```python
from build123d import *

# Parameters (mm, degrees)
SKETCH_1_W               = 35
SKETCH_1_H               = 40
EXTRUDE_1_DEPTH          = 2
SKETCH_2_R               = 1.6
CUT_EXTRUDE_1_DEPTH      = 2
SKETCH_3_W               = 6
SKETCH_3_H               = 6
EXTRUDE_2_DEPTH          = 22
SKETCH_4_W               = 32
SKETCH_4_H               = 32
SKETCH_4_R               = 1.65
EXTRUDE_3_DEPTH          = 3
SKETCH_5_W               = 2.5
SKETCH_5_H               = 22
EXTRUDE_4_DEPTH          = 3
PATTERN_CIRCULAR_1_COUNT = 4


with BuildPart() as part:
    # 草图1 → 凸台-拉伸1 (new body)
    with BuildSketch(Plane(origin=(0, 0, 0), x_dir=(1, 0, 0), z_dir=(0, 1, 0))):
        Rectangle(SKETCH_1_W, SKETCH_1_H)
    extrude(amount=EXTRUDE_1_DEPTH)

    # 草图2 → 切除-拉伸1 (cut)
    with BuildSketch(Plane(origin=(0, 2, 0), x_dir=(1, 0, 0), z_dir=(0, 1, 0))):
        with Locations(Location((-12.5, 15, 0), (0, 0, 270))):
            Circle(SKETCH_2_R)
        with Locations(Location((12.5, 15, 0), (0, 0, 90))):
            Circle(SKETCH_2_R)
        with Locations(Location((12.5, -15, 0), (0, 0, 270))):
            Circle(SKETCH_2_R)
        with Locations(Location((-12.5, -15, 0), (0, 0, 90))):
            Circle(SKETCH_2_R)
    extrude(amount=-CUT_EXTRUDE_1_DEPTH, mode=Mode.SUBTRACT)

    # 草图3 → 凸台-拉伸2 (add)
    with BuildSketch(Plane(origin=(0, 2, 0), x_dir=(1, 0, 0), z_dir=(0, 1, 0))):
        Rectangle(SKETCH_3_W, SKETCH_3_H)
    extrude(amount=EXTRUDE_2_DEPTH)

    # 草图4 → 凸台-拉伸3 (add)
    with BuildSketch(Plane(origin=(0, 24, 0), x_dir=(1, 0, 0), z_dir=(0, 1, 0))):
        Rectangle(SKETCH_4_W, SKETCH_4_H)
        with Locations(Location((-7.78, 7.78, 0), (0, 0, 270))):
            Circle(SKETCH_4_R, mode=Mode.SUBTRACT)
        with Locations(Location((7.78, 7.78, 0), (0, 0, 90))):
            Circle(SKETCH_4_R, mode=Mode.SUBTRACT)
        with Locations(Location((7.78, -7.78, 0), (0, 0, 270))):
            Circle(SKETCH_4_R, mode=Mode.SUBTRACT)
        with Locations(Location((-7.78, -7.78, 0), (0, 0, 90))):
            Circle(SKETCH_4_R, mode=Mode.SUBTRACT)
    extrude(amount=EXTRUDE_3_DEPTH)

    # 草图5 → 凸台-拉伸4 (add)
    with BuildSketch(Plane.XY.offset(3)):
        with Locations((0, 13)):
            Rectangle(SKETCH_5_W, SKETCH_5_H)
    extrude_4 = extrude(amount=EXTRUDE_4_DEPTH)

    # 阵列(圆周)1: 凸台-拉伸4 ×4 about axis
    pattern_circular_1_axis = Axis((0, 0, 0), (0, 1, 0))
    for i in range(1, PATTERN_CIRCULAR_1_COUNT):
        add(extrude_4.rotate(pattern_circular_1_axis, i * 360 / PATTERN_CIRCULAR_1_COUNT))


solid = part.part
```
Geometry check sheet. Reference: the model listing, model coordinates, mm. A direction names the side the tool comes from. Coordinates: 2 decimals unless noted, no trailing zeros. Order: outer loops, then holes, each group sorted by start corner. A loop starts at its lowest first (then second) coordinate and runs counter-clockwise, first axis right, second up. Notation, with made-up numbers: M 42,-34.75 L 71,-34.75 A29 cw 71,-5.75 Z; hole C 15,-8.5 d3. An arc over 180 degrees is marked long. One line per question, with ' | ' between items. Start each with the question number.
Item 1: Set-up check for faces 4 (the flat face through (-4, 13, 1.25)), 5 (the flat face through (-3, 13, -2)), 6 (the flat face through (1.25, 13, 4)), 7 (the cylindrical face through (12.43, 1.01, -13.4)), 8 (the cylindrical face through (-9.4, 25.5, -8.1)): record each of +Z, -Z, +X, -X, +Y, -Y from which the full face is reachable in a straight line by a thin tool's end or side.
Item 2: Gauge pin test, flat ends, axial feed: pin 1 (0.9 mm diameter, centred on y = 18.5, z = 2.5, fed in from +X); pin 2 (0.9 mm diameter, centred on x = 2.5, y = 14.5, fed in from -Z); pin 3 (1.5 mm diameter, centred on x = -5, y = 25, fed in from -Z). Record the tip position at first contact, or that the pin passes through.
Item 3: Cross-section at A-A on z = -12. Enter the section's corners in (x, y).
Item 4: Cross-section at C-C on z = -7.78. Enter the section's corners in (x, y).
Item 5: Cross-section at D-D on x = -5.5. Enter the section's corners in (y, z).
Item 6: Cross-section at B-B on x = -12.5. Enter the section's corners in (y, z).
Item 7: Draft check along X on faces 1 (the cylindrical face through (-13.58, 1.01, 16.18)), 2 (the flat face through (-4, 13, -1.25)), 3 (the flat face through (3, 13, -2)). Enter one of: pulls with the +X half, pulls with the -X half, needs draft (parallel to the pull), parting line crosses it, or undercut.
Item 8: Material ranges on L1, parallel to X at y = 25.85, z = 7.78; L2, parallel to X at y = 0.6, z = 15; L3, parallel to Y at x = -1, z = -7, recorded low to high. Write a range as [from, to].
Findings:
1) face 4: +Z, -X | face 5: -Z, -X | face 6: +Z, +X | face 7: -Y | face 8: +Y
2) pin 1: stops at x = 3 | pin 2: stops at z = -3 | pin 3: stops at z = -16
3) outline: M -17.5,0 L 17.5,0 L 17.5,2 L -17.5,2 Z; M -16,24 L 16,24 L 16,27 L -16,27 Z
4) outline: M -17.5,0 L 17.5,0 L 17.5,2 L -17.5,2 Z; M -16,24 L -9.43,24 L -9.43,27 L -16,27 Z; M -6.13,24 L 6.13,24 L 6.13,27 L -6.13,27 Z; M 9.43,24 L 16,24 L 16,27 L 9.43,27 Z
5) outline: M 0,-20 L 2,-20 L 2,-1.25 L 24,-1.25 L 24,-16 L 27,-16 L 27,16 L 24,16 L 24,1.25 L 2,1.25 L 2,20 L 0,20 Z
6) outline: M 0,-20 L 2,-20 L 2,-16.6 L 0,-16.6 Z; M 0,-13.4 L 2,-13.4 L 2,13.4 L 0,13.4 Z; M 0,16.6 L 2,16.6 L 2,20 L 0,20 Z; M 24,-16 L 27,-16 L 27,16 L 24,16 Z
7) face 1: undercut | face 2: needs draft | face 3: pulls with the +X half
8) L1: x = [-16, -9.43], [-6.13, 6.13], [9.43, 16] | L2: x = [-17.5, -14.1], [-10.9, 10.9], [14.1, 17.5] | L3: y = [0, 2], [24, 27]
